from build123d import *

# Parameters (mm, degrees)
BOSS_EXTRU_1_DEPTH      = 2.400000114
ESQUISSE9_W             = 36.19999811
ESQUISSE9_H             = 2.400000114
BOSS_EXTRU_2_DEPTH      = 5
ESQUISSE14_R            = 7.502289609
ENL_V_MAT_EXTRU_1_DEPTH = 72.750046163
ENL_V_MAT_EXTRU_2_DEPTH = 72.750046163
ESQUISSE25_R            = 1.252758793
ENL_V_MAT_EXTRU_3_DEPTH = 72.750046163
ESQUISSE28_R            = 2.406964412
BOSS_EXTRU_3_DEPTH      = 2.9
SKETCH1_R               = 7.502289609
BOSS_EXTRUDE1_DEPTH     = 8
CUT_EXTRUDE2_START      = -6
CUT_EXTRUDE2_DEPTH      = 6


with BuildPart() as part:
    # Esquisse4 → Boss.-Extru.1 (new body)
    with BuildSketch(Plane.XY.offset(2.400000114)):
        with BuildLine():
            Line((-20.100001246, -24.634756148), (-48.900358379, 4.499999806))
            Line((-48.900358379, 4.499999806), (-60.405611992, 4.499999806))
            ThreePointArc((-60.405611992, 4.499999806), (-65.300002694, -0.500000082), (-60.405611992, -5.49999997))
            Line((-60.405611992, -5.49999997), (-56.299999356, -5.49999997))
            Line((-56.299999356, -5.49999997), (-56.299999356, -24.634756148))
            Line((-56.299999356, -24.634756148), (-20.100001246, -24.634756148))
        make_face()
    extrude(amount=-BOSS_EXTRU_1_DEPTH)

    # Esquisse9 → Boss.-Extru.2 (add)
    with BuildSketch(Plane(origin=(0, -24.634756148, 0), x_dir=(-1, 0, 0), z_dir=(0, -1, 0))):
        with Locations((38.200000301, -1.200000057)):
            Rectangle(ESQUISSE9_W, ESQUISSE9_H)
    extrude(amount=BOSS_EXTRU_2_DEPTH)

    # Esquisse14 → Enlèv. mat.-Extru.1 (cut, through all)
    with BuildSketch(Plane.XY.offset(2.400000114)):
        with Locations((-43.700002134, -16.999939794)):
            Circle(ESQUISSE14_R)
    extrude(amount=-ENL_V_MAT_EXTRU_1_DEPTH, mode=Mode.SUBTRACT)

    # Esquisse19 → Enlèv. mat.-Extru.2 (cut, through all)
    with BuildSketch(Plane.XY.offset(2.400000114)):
        Polygon((-26.350000873, -28.503000736), (-25.724001229, -28.334999457), (-25.264998898, -27.875998989), (-25.096999481, -27.249999344), (-25.264998898, -26.6239997), (-25.724001229, -26.165001094), (-26.350000873, -25.998000056), (-26.976000518, -26.165001094), (-27.434999123, -26.6239997), (-27.602000162, -27.249999344), (-27.434999123, -27.875998989), (-26.976000518, -28.334999457), align=None)
    extrude(amount=-ENL_V_MAT_EXTRU_2_DEPTH, mode=Mode.SUBTRACT)

    # Esquisse25 → Enlèv. mat.-Extru.3 (cut, through all)
    with BuildSketch(Plane(origin=(0, 0, 0), x_dir=(-1, 0, 0), z_dir=(0, 0, -1))):
        with Locations((50.350001082, -27.250241944)):
            Circle(ESQUISSE25_R)
    extrude(amount=-ENL_V_MAT_EXTRU_3_DEPTH, mode=Mode.SUBTRACT)

    # Esquisse28 → Boss.-Extru.3 (add)
    with BuildSketch(Plane.XY.offset(2.400000114)):
        with Locations((-60.267728087, -0.4991006)):
            Circle(ESQUISSE28_R)
    extrude(amount=BOSS_EXTRU_3_DEPTH)

    # Sketch1 → Boss-Extrude1 (add)
    with BuildSketch(Plane.XY.offset(2.400000114)):
        with BuildLine():
            Line((-56.299999356, -24.634756148), (-56.299999356, -5.49999997))
            Line((-56.299999356, -5.49999997), (-60.405611992, -5.49999997))
            ThreePointArc((-60.405611992, -5.49999997), (-65.40561188, -0.500000082), (-60.405611992, 4.499999806))
            Line((-60.405611992, 4.499999806), (-48.900358379, 4.499999806))
            Line((-48.900358379, 4.499999806), (-20.100001246, -24.634756148))
            Line((-20.100001246, -24.634756148), (-56.299999356, -24.634756148))
        make_face()
        with Locations((-43.700002134, -16.999939794)):
            Circle(SKETCH1_R, mode=Mode.SUBTRACT)
    extrude(amount=-BOSS_EXTRUDE1_DEPTH)

    # Sketch3 → Cut-Extrude2 (cut)
    with BuildSketch(Plane(origin=(0, 0, -5.599999886), x_dir=(-1, 0, 0), z_dir=(0, 0, -1)).offset(CUT_EXTRUDE2_START)):
        with BuildLine():
            Line((56.299999356, -8.9560628), (56.299999356, -5.49999997))
            Line((56.299999356, -5.49999997), (60.405611992, -5.49999997))
            ThreePointArc((60.405611992, -5.49999997), (65.40561188, -0.500000082), (60.405611992, 4.499999806))
            Line((60.405611992, 4.499999806), (48.900358379, 4.499999806))
            Line((48.900358379, 4.499999806), (35.598739883, -8.9560628))
            Line((35.598739883, -8.9560628), (56.299999356, -8.9560628))
        make_face()
    extrude(amount=CUT_EXTRUDE2_DEPTH, mode=Mode.SUBTRACT)


solid = part.part
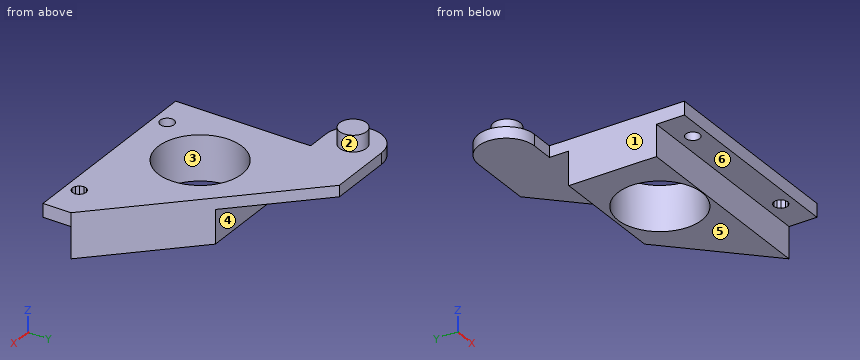
Geometry: final body of the model. Coordinates: model frame, mm. Face numbers are marked on the shaded views. A direction names the side the tool comes from. Round coordinates to 2 decimals unless told otherwise and drop trailing zeros. Order: outer loops, then holes, each group sorted by start corner. A loop starts at its lowest first (then second) coordinate and runs counter-clockwise, first axis right, second up. Notation, with made-up numbers: (11, 62.5) -> (68, 62.5) arc R33 ccw to (68, 91.5) -> close; hole circle Ø3 at (22, 82). An arc over 180 degrees is marked (long way). Put each result on its own line as item: value. Start each with the question number.
Q1. Section C-C on x = -61. Return the cut outline in (y, z).
Q2. Pull-direction query (X, two-part tool) for the marked faces 1, 2 and 3; classes: +X half, -X half, draft (parallel to the pull), parting line (faces both ways), or undercut.
Q3. Section B-B on z = 1.25. Return the cut outline in (x, y) (3 decimals), and give its area (3 significant figures).
Q4. Line query: probe 1 along Z at (x, y) = (-50, -0.5); probe 2 along Z at (x, y) = (-43, -27); probe 3 along Y at (x, z) = (-39, -4.5). Output: solid intervals per line, ascending.
Q5. Section A-A on y = -10. Return the cut outline in (x, z), and give its area (3 significant figures).
Q6. Section D-D on y = 0. Return the cut outline in (x, z), and give its area (3 significant figures).
Q7. Reachability of the marked faces 4, 5 and 6 from +Z, -Z, +X, -X, +Y, -Y: full face, straight path, thin tool, end or side. Return the list, or none.
Q8. First-contact query: pin 1 (17 mm diameter, centred on x = -48, y = -16, fed in from +Z); pin 2 (2.5 mm diameter, centred on x = -39.5, y = -27.5, fed in from -Z); pin 3 (0.6 mm diameter, centred on x = -57.5, z = 1.5, fed in from -Y). Flat tips, straight axial feed; report the tip coordinate or a pass-through.
Ans:
1. outline: (-5.46, 0.4) -> (4.46, 0.4) -> (4.46, 2.4) -> (1.79, 2.4) -> (1.79, 5.3) -> (-2.79, 5.3) -> (-2.79, 2.4) -> (-5.46, 2.4) -> close
2. face 1: -X half
2. face 2: parting line
2. face 3: undercut
3. outline: (-60.406, -5.5) -> (-56.3, -5.5) -> (-56.3, -29.635) -> (-20.1, -29.635) -> (-20.1, -24.635) -> (-48.9, 4.5) -> (-60.406, 4.5) arc R5 ccw to start; hole circle Ø2.506 at (-50.35, -27.25); hole circle Ø15.005 at (-43.7, -17); hole (-27.602, -27.25) -> (-27.435, -27.876) -> (-26.976, -28.335) -> (-26.35, -28.503) -> (-25.724, -28.335) -> (-25.265, -27.876) -> (-25.097, -27.25) -> (-25.265, -26.624) -> (-25.724, -26.165) -> (-26.35, -25.998) -> (-26.976, -26.165) -> (-27.435, -26.624) -> close
3. area: 710 mm2
4. probe 1: z = 0.4 to 2.4
4. probe 2: z = 0 to 2.4
4. probe 3: y = -24.63 to -22.85, -11.15 to -8.96
5. outline: (-56.3, -5.6) -> (-46.4, -5.6) -> (-46.4, 2.4) -> (-56.3, 2.4) -> close; (-41, -5.6) -> (-34.57, -5.6) -> (-34.57, 2.4) -> (-41, 2.4) -> close
5. area: 131 mm2
6. outline: (-65.38, 0.4) -> (-44.45, 0.4) -> (-44.45, 2.4) -> (-57.91, 2.4) -> (-57.91, 5.3) -> (-62.62, 5.3) -> (-62.62, 2.4) -> (-65.38, 2.4) -> close
6. area: 55.5 mm2
7. face 4: -Z, +X, -X, +Y
7. face 5: -Z, +X, -X, +Y, -Y
7. face 6: -Z, +X, -X, -Y
8. pin 1: stops at z = 2.4
8. pin 2: stops at z = 0
8. pin 3: stops at y = -5.5
